CAD build for the part. Positions are in the model's coordinates, mm. A direction names the side the tool comes from. Coordinates: 2 decimals unless noted, no trailing zeros. Loops run counter-clockwise (first coordinate to the right, second up) from the corner with the lowest first, then second, coordinate; pieces in that order, holes last.
1) Saw through at A-A, the plane y = 10.1. Write the cut outline in (x, z), and give its area (3 significant figures).
2) Saw through at B-B, the plane y = 4.25. Write the cut outline in (x, z).
3) Pin check, flat tips, straight feed: pin 1 Ø1.4 at (y, z) = (2, 0) entering from -X; pin 2 Ø4 at (y, z) = (-4, -3) entering from -X; pin 3 Ø2 at (y, z) = (-4.5, -1) entering from -X. Stop position of each tip, or through.
4) Two-plate mould, pull along Y, no slides. Class faces 5 (the flat face through (0, 12.2, 0)), 6 (the cylindrical face through (3.905, -2.028, -0.867)), 7 (the flat face through (4, 0, 2)), 8 (the flat face through (-2.8, 2, 0)): +Y half, -Y half, draft (parallel to the pull), parting line (faces both ways), or undercut.
5) Which spindle directions (+Z, -Z, +X, -X, +Y, -Y) get a long thin tool onto all of the face, cutting with end or side? Do faces 1 (the flat face through (-2, -4, 0)), 2 (the cylindrical face through (-4.861, 1.121, -0.195)), 3 (the flat face through (-1, -5, 0)), 4 (the flat face through (4, 4, 2)). Say none if no direction does.
6) Wall check: line 1 along Y through (x, z) = (-5.5, -0.25); line 2 along X through (y, z) = (0.5, -0.25); line 3 along Y through (x, z) = (6.25, -3.5). Give the ranges that are in metal, low to high.
```python
from build123d import *

# Parameters (mm, degrees)
SKETCH_1_R          = 7.8
EXTRUDE_1_DEPTH     = 4
SKETCH_2_R          = 4
EXTRUDE_2_DEPTH     = 8.2
SWEEP_1_PROFILE_R   = 1
SKETCH_10_R         = 0.9
CUT_EXTRUDE_3_DEPTH = 19.679400419
EXTRUDE_START       = 4
SKETCH_12_R         = 4
EXTRUDE_3_DEPTH     = 4
EXTRUDE_4_DEPTH     = 2
SKETCH_14_R         = 0.9
CUT_EXTRUDE_4_DEPTH = 5
SKETCH_15_W         = 7.770297698
SKETCH_15_H         = 4
CUT_EXTRUDE_5_DEPTH = 0.5


with BuildPart() as part:
    # 草图1 → 凸台-拉伸1 (new body)
    with BuildSketch(Plane(origin=(0, 0, 0), x_dir=(1, 0, 0), z_dir=(0, 1, 0))):
        with Locations(Location((0, 0, 0), (0, 0, 270))):
            Circle(SKETCH_1_R)
    extrude(amount=EXTRUDE_1_DEPTH)

    # 草图2 → 凸台-拉伸2 (add)
    with BuildSketch(Plane(origin=(0, 4, 0), x_dir=(1, 0, 0), z_dir=(0, 1, 0))):
        with Locations(Location((0, 0, 0), (0, 0, 270))):
            Circle(SKETCH_2_R)
    extrude(amount=EXTRUDE_2_DEPTH)

    # 切除-扫描1: sweep along a path in 草图5
    with BuildLine(Plane(origin=(0, 2, 0), x_dir=(1, 0, 0), z_dir=(0, 1, 0))) as sweep_1_path:
        CenterArc((0, 0), 7.3, 0, 360)
    # 切除-扫描1 profile (on start of the path) → 切除-扫描1 (sweep, cut)
    with BuildSketch(Plane(origin=(7.3, 2, 0), x_dir=(-1, 0, 0), z_dir=(0, 0, -1))):
        Circle(SWEEP_1_PROFILE_R)
    sweep(path=sweep_1_path.line, mode=Mode.SUBTRACT)

    # 草图10 → 切除-拉伸3 (cut, through all)
    with BuildSketch(Plane(origin=(0, 0, -4), x_dir=(-1, 0, 0), z_dir=(0, 0, -1))):
        with Locations(Location((0, 10.1, 0), (0, 0, 89.999999955))):
            Circle(SKETCH_10_R)
    extrude(amount=-CUT_EXTRUDE_3_DEPTH, mode=Mode.SUBTRACT)

    # 草图12 → 凸台-拉伸3 (add)
    with BuildSketch(Plane.XZ.offset(EXTRUDE_START)):
        with Locations(Location((0, 0, 0), (0, 0, 90))):
            Circle(SKETCH_12_R)
    extrude(amount=-EXTRUDE_3_DEPTH)

    # 草图13 → 凸台-拉伸4 (add)
    with BuildSketch(Plane.XZ.offset(4)):
        with BuildLine():
            ThreePointArc((2, 0), (1, 1.732050808), (-1, 1.732050808))
            Line((-1, 1.732050808), (-1, -1.732050808))
            ThreePointArc((-1, -1.732050808), (1, -1.732050808), (2, 0))
        make_face()
    extrude(amount=EXTRUDE_4_DEPTH)

    # 草图14 → 切除-拉伸4 (cut)
    with BuildSketch(Plane.ZY.offset(7.8)):
        with Locations((0, 2)):
            Circle(SKETCH_14_R)
    extrude(amount=-CUT_EXTRUDE_4_DEPTH, mode=Mode.SUBTRACT)

    # 草图15 → 切除-拉伸5 (cut)
    with BuildSketch(Plane.ZY.offset(7.8)):
        with Locations((0.165386451, 2)):
            Rectangle(SKETCH_15_W, SKETCH_15_H)
    extrude(amount=-CUT_EXTRUDE_5_DEPTH, mode=Mode.SUBTRACT)


solid = part.part
```
Data:
1. outline: (-0.9, -3.9) - (-0.9, 3.9) arc R4 ccw to start; (0.9, -3.9) arc R4 ccw to (0.9, 3.9) - close
1. area: 36.0 mm2
2. outline: circle Ø8 at (0, 0)
3. pin 1: stops at x = -2.8
3. pin 2: stops at x = -3.87
3. pin 3: stops at x = -4
4. face 5: +Y half
4. face 6: draft
4. face 7: -Y half
4. face 8: undercut
5. face 1: -Y
5. face 2: -X
5. face 3: +Z, -Z, -X, -Y
5. face 4: +Y
6. line 1: y = 0 to 1.14, 2.86 to 4
6. line 2: x = -7.3 to 7.8
6. line 3: y = 0 to 1.01, 2.99 to 4
